Check sheet for the modelled part. Datum: model origin and axes. Units: mm. Face numbers are marked on the shaded views. A direction names the side the tool comes from. Give positions to 0.01 mm unless a question says otherwise; leave off trailing zeros. Order: outer loops, then holes, each group sorted by start corner. A loop starts at its lowest first (then second) coordinate and runs counter-clockwise, first axis right, second up.
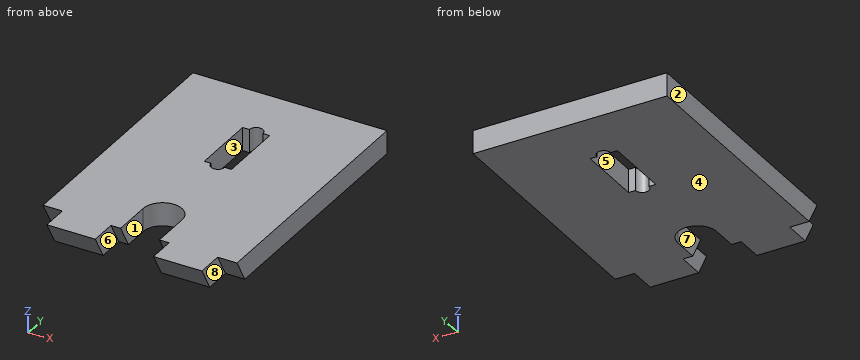
Autodesk Inventor part; units mm, degrees
ref_plane "YZ Plane" through (0, 0, 0) normal (1, 0, 0) x (0, 1, 0)
ref_plane "XZ Plane" through (0, 0, 0) normal (0, 1, 0) x (-1, 0, 0)
ref_plane "XY Plane" through (0, 0, 0) normal (0, 0, 1) x (1, 0, 0)
sketch "Sketch1" plane through (0, 0, 0) normal (0, 0, 1) x (1, 0, 0)
  line L0 (25, -30) -> (-25, -30)
  line L1 (-25, -30) -> (-25, 30)
  line L2 (-25, 30) -> (25, 30)
  line L3 (25, 30) -> (25, -30)
  line L4 (-25, 0) -> (25, 0) construction
  point P0 (0, 0)
  point P1 (0, 0)
  dimension "d0" = 50
  dimension "d1" = 60
extrude "Extrusion1" add sketch "Sketch1" along normal blind 6
sketch "Sketch2" plane through (-25, -30, 0) normal (-1, 0, 0) x (0, 0, 1)
  line L0 (0, 0) -> (6, 0)
  line L1 (6, -3.4641) -> (-173.2051, 100) construction
  line L2 (0, 0) -> (6, -3.4641)
  line L3 (6, -3.4641) -> (6, 0)
  point P0 (0, 30)
extrude "Extrusion2" add sketch "Sketch2" against normal blind 50
sketch "Sketch4" plane through (-25, 30, 0) normal (-1, 0, 0) x (0, 0, 1)
  line L0 (6, -63.4641) -> (6, 0)
  line L1 (0, -60) -> (0, 0)
  line L2 (0, -60) -> (6, -63.4641)
  line L3 (6, -56.5359) -> (-167.2051, 43.4641) construction
  line L4 (0, -53.0718) -> (6, -56.5359)
  point P0 (0, -30)
extrude "Extrusion3" cut sketch "Sketch4" against normal blind 5
sketch "Sketch7" plane through (0, 0, 0) normal (1, 0, 0) x (0, 1, 0)
  line L0 (-23.0718, 0) -> (-30, 0) construction
  line L1 (70, -173.2051) -> (-33.4641, 6) construction
  line L2 (-33.4641, 6) -> (-26.5359, 6) construction
  line L3 (-26.5359, 6) -> (73.4641, -167.2051) construction
  line L4 (-33.4641, 6) -> (-30, 0)
  line L5 (-23.0718, 0) -> (-30, 0)
  line L6 (-33.4641, 6) -> (-26.5359, 6)
  line L7 (-26.5359, 6) -> (-23.0718, 0)
  point P0 (0, 0)
extrude "Extrusion6" cut sketch "Sketch7" along normal mid plane 15
mirror "Mirror1" about plane through (0, 0, 0) normal (1, 0, 0) of "Extrusion3"
sketch "Sketch8" plane through (0, 0, 6) normal (0, 0, 1) x (1, 0, 0)
  line L0 (-7.5, -26.5359) -> (7.5, -26.5359)
  line L1 (-5, -26.5359) -> (5, -26.5359)
  line L2 (5, -26.5359) -> (5, -16.5359)
  line L3 (5, -16.5359) -> (-5, -16.5359) construction
  line L4 (-5, -16.5359) -> (-5, -26.5359)
  arc A0 (5, -16.5359) -> (-5, -16.5359) centre (0, -16.5359) ccw
  point P0 (0, 0)
  point P1 (0, -26.5359)
  dimension "d23" = 10
  dimension "d24" = 10
extrude "Extrusion7" cut sketch "Sketch8" against normal up to next
thicken "Thicken1" operation add thickness 10 both sides no extend neighbours yes toward (0, 1, 0) faces at (-8.3333, 30, 2)
sketch "Sketch11" plane through (0, 0, 6) normal (0, 0, 1) x (1, 0, 0)
  line L0 (-25, 40) -> (25, 40)
  line L1 (-3.5, 25) -> (3.5, 25)
  line L2 (3.5, 25) -> (3.5, 8)
  line L3 (3.5, 8) -> (-3.5, 8)
  line L4 (-3.5, 8) -> (-3.5, 25)
  line L5 (0, 40) -> (0, 0) construction
  line L6 (0, 40) -> (0, 0) construction
  circle A0 centre (0, 25) radius 1.75
  circle A1 centre (0, 8) radius 1.75
  dimension "d40" = 7
  dimension "d41" = 17
  dimension "d42" = 15
  dimension "d43" = 3.5
  dimension "d44" = 3.5
extrude "Extrusion10" cut sketch "Sketch11" against normal up to next
equation "\"d44\" = d43"
properties part number "TRIANGLESHORTLEG"
(1) Cross-section at C-C on z = 4.25. Enter the section's corners in (x, y), then the cut area to 3 significant figures.
Response values:
outline: (-25, -25.53) - (-20, -25.53) - (-20, -32.45) - (-7.5, -32.45) - (-7.5, -25.53) - (-5, -25.53) - (-5, -16.54) arc R5 cw to (5, -16.54) - (5, -25.53) - (7.5, -25.53) - (7.5, -32.45) - (20, -32.45) - (20, -25.53) - (25, -25.53) - (25, 40) - (-25, 40) - close; hole (-3.5, 8) - (-1.75, 8) arc R1.75 ccw to (1.75, 8) - (3.5, 8) - (3.5, 25) - (1.75, 25) arc R1.75 ccw to (-1.75, 25) - (-3.5, 25) - close
area: 3,190 mm2
(2) Cross-section at B-B on x = 0. Enter the section's corners in (y, z), then the cut area to 3 significant figures.
Response values:
outline: (-11.54, 0) - (6.25, 0) - (6.25, 6) - (-11.54, 6) - close; (26.75, 0) - (40, 0) - (40, 6) - (26.75, 6) - close
area: 186 mm2
(3) Material ranges on L1, parallel to X at y = 16, z = 3.5; L2, parallel to Y at x = 0, z = 5.25; L3, parallel to Y at x = -6, z = 4, recorded low to high.
Response values:
L1: x = -25 to -3.5, 3.5 to 25
L2: y = -11.54 to 6.25, 26.75 to 40
L3: y = -25.38 to 40
(4) Cross-section at D-D on x = 16. Enter the section's corners in (y, z).
Response values:
outline: (-33.46, 6) - (-30, 0) - (40, 0) - (40, 6) - close
(5) Set-up check for the marked faces 5, 6, 7 and 8: record each of +Z, -Z, +X, -X, +Y, -Y from which the full face is reachable in a straight line by a thin tool's end or side.
Response values:
face 5: +Z, -Z
face 6: -Z, -Y
face 7: +Z, -Z, -Y
face 8: -Z, +X, -Y
(6) Gauge pin test, flat ends, axial feed: pin 1 Ø1.5 at (x, z) = (-4.5, 4.5) entering from -Y; pin 2 Ø1.8 at (y, z) = (-29, 1.5) entering from -X; pin 3 Ø0.5 at (x, z) = (-2.5, 2) entering from -Y. Record the tip position at first contact, or that the pin passes through.
Response values:
pin 1: stops at y = -25.99
pin 2: stops at x = -20
pin 3: stops at y = -12.36
(7) Release check for a two-part mould opening along X. For the marked faces 1, 2, 3 and 4 record: released by +X, released by -X, zero draft, split by the parting line, or undercut.
Response values:
face 1: undercut
face 2: released by -X
face 3: undercut
face 4: zero draft
(8) Cross-section at A-A on y = 18. Enter the section's corners in (x, z).
Response values:
outline: (-25, 0) - (-3.5, 0) - (-3.5, 6) - (-25, 6) - close; (3.5, 0) - (25, 0) - (25, 6) - (3.5, 6) - close
